The model under review builds one solid part; all positions refer to its coordinate system, in mm. Face numbers are marked on the shaded views. Round coordinates to 2 decimals unless told otherwise and drop trailing zeros. Order: outer loops, then holes, each group sorted by start corner. A loop starts at its lowest first (then second) coordinate and runs counter-clockwise, first axis right, second up. Notation, with made-up numbers: M -1.5,-36 L 17.5,-36 A18 ccw 17.5,-5 Z; hole C 63,36 d5. An arc over 180 degrees is marked long. Use a Markdown table: item, result. Add a question column.
1. Consider section C-C on y = 0.15. State the section outline as (x, z) points (3 decimals).
2. Consider section B-B on z = 1.25. State the section outline as (x, y) points.
3. Consider section A-A on x = 1. State the section outline as (y, z) points, then the cut area to 3 significant figures.
4. To check wall thickness, follow probe 1 along X at (y, z) = (0.85, 0) (3 decimals); probe 2 along X at (y, z) = (0.8, 1.25); probe 3 along Z at (x, y) = (-1.75, 0.1). State the ranges of each line that lie inside material, in increasing order.
5. Consider section D-D on z = 2.5. State the section outline as (x, y) points.
6. The part is to be moulded in two halves that separate along Z. For the marked faces 1, 2 and 3, say which applies: +Z half, -Z half, draft (parallel to the pull), parting line (faces both ways), or undercut.
from build123d import *

# Parameters (mm, degrees)
SKETCH1_R               = 3.175
BOSS_EXTRUDE1_DEPTH     = 1.5875
CUT_EXTRUDE2_DEPTH      = 5.7625
CUT_EXTRUDE2_DEPTH_BACK = 5.7625
CUT_EXTRUDE3_DEPTH      = 5.7625
CUT_EXTRUDE3_DEPTH_BACK = 5.7625
SKETCH3_R               = 2.286


with BuildPart() as part:
    # Sketch1 → Boss-Extrude1 (new body)
    with BuildSketch(Plane(origin=(0, 0, 0), x_dir=(1, 0, 0), z_dir=(0, 1, 0))):
        with Locations(Location((0, 0, 0), (0, 0, 270))):
            Circle(SKETCH1_R)
    extrude(amount=BOSS_EXTRUDE1_DEPTH)

    # Sketch2 → Cut-Extrude2 (cut, two sides: drawn at the far end of the back side and taken through both)
    with BuildSketch(Plane(origin=(0, 0, 0), x_dir=(0, 0, -1), z_dir=(1, 0, 0)).offset(-CUT_EXTRUDE2_DEPTH_BACK)):
        Polygon((3.175, 1.5875), (-3.175, 0.503215254), (-3.175, 1.5875), align=None)
    extrude(amount=CUT_EXTRUDE2_DEPTH + CUT_EXTRUDE2_DEPTH_BACK, mode=Mode.SUBTRACT)

    # Sketch3 → Cut-Extrude3 (cut, two sides: drawn at the far end of the back side and taken through both)
    with BuildSketch(Plane.XZ.offset(-CUT_EXTRUDE3_DEPTH_BACK)):
        with Locations(Location((0, 0, 0), (0, 0, 90))):
            Circle(SKETCH3_R)
    extrude(amount=CUT_EXTRUDE3_DEPTH + CUT_EXTRUDE3_DEPTH_BACK, mode=Mode.SUBTRACT)


solid = part.part
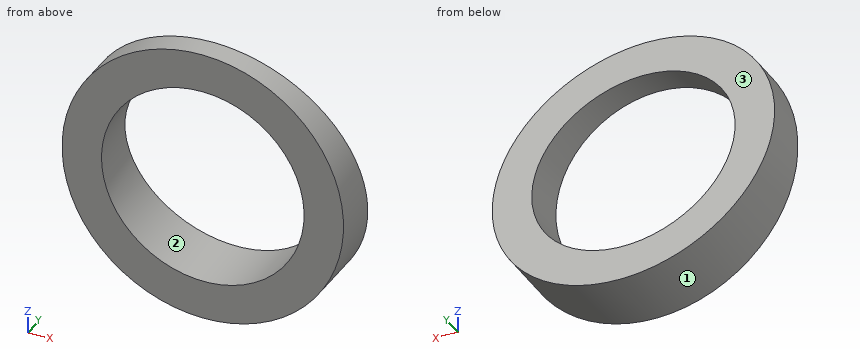
Answer block:
| question | item | result |
|---|---|---|
| 1 | outline | C 0,0 d6.35; hole C 0,0 d4.572 |
| 2 | outline | M -2.92,0 L -1.91,0 L -1.91,0.83 L -2.92,0.83 Z; M 1.91,0 L 2.92,0 L 2.92,0.83 L 1.91,0.83 Z |
| 3 | outline | M 0,-3.01 L 1.56,-3.01 L 1.4,-2.06 L 0,-2.06 Z; M 0,2.06 L 0.69,2.06 L 0.53,3.01 L 0,3.01 Z |
| 3 | area | 2.00 mm^2 |
| 4 | probe 1 | -3.175 to -2.286, 2.286 to 3.175 |
| 4 | probe 2 | -2.92 to -1.91, 1.91 to 2.92 |
| 4 | probe 3 | -2.65 to -1.47, 1.47 to 2.65 |
| 5 | outline | M -1.96,0 L 1.96,0 L 1.96,0.62 L -1.96,0.62 Z |
| 6 | face 1 | parting line |
| 6 | face 2 | undercut |
| 6 | face 3 | +Z half |
